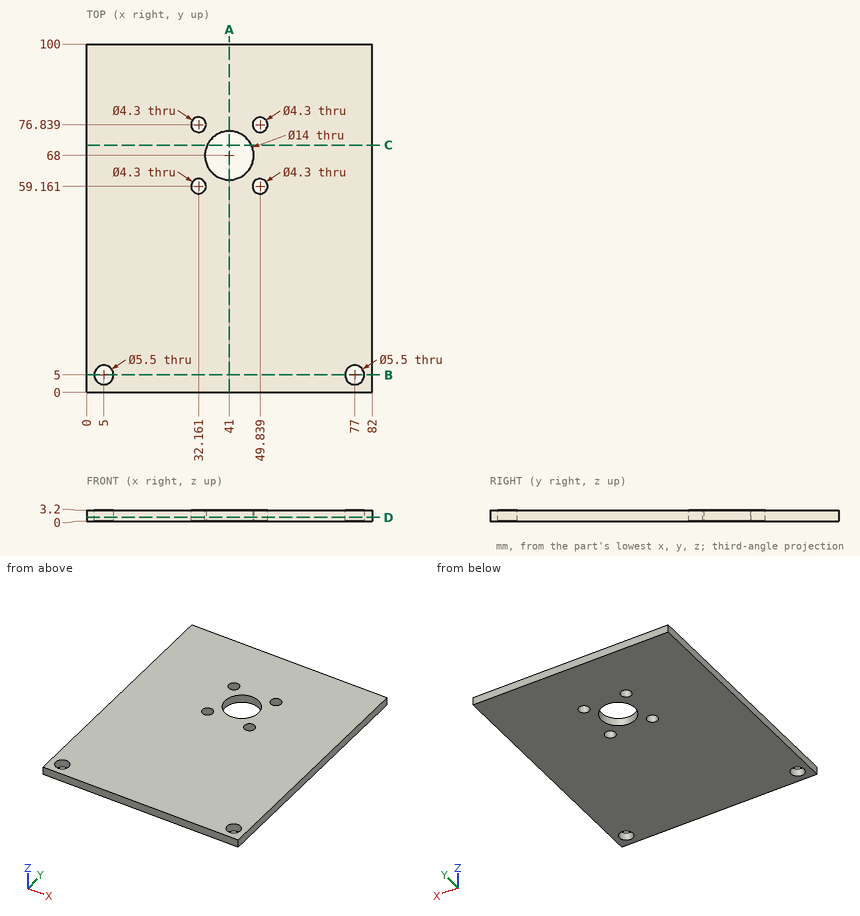
Can you work these out from the drawing? Everything is in mm from the part's minimum corner. Give positions to 0.01 mm unless a question says otherwise; leave off trailing zeros. Order: outer loops, then holes, each group sorted by start corner. A loop starts at its lowest first (then second) coordinate and runs counter-clockwise, first axis right, second up. Notation, with made-up numbers: (-38, 82.25) -> (-16, 82.25) arc R27 ccw to (-16, 114.25) -> close; hole circle Ø2 at (84.25, 34.25). An arc over 180 degrees is marked (long way). Return JSON: item names as keys, results as strings.
1. I need wall thicknesses on line 1 (X direction, y = 75.5, z = 2.25); line 2 (X direction, y = 6.5, z = 2.7) (1 decimal); line 3 (Y direction, x = 41, z = 1.5). Which ranges of each line are inside material? Lowest first, please. Write a range as from..to.
Answer list:
{"line 1": "x = 0..30.48, 33.84..48.16, 51.52..82", "line 2": "x = 0..2.7, 7.3..74.7, 79.3..82", "line 3": "y = 0..61, 75..100"}
2. Imagine slicing it at B-B on y = 5. List the corners of the cut face in (x, z) for me.
Answer list:
{"outline": "(0, 0) -> (2.25, 0) -> (2.25, 3.2) -> (0, 3.2) -> close; (7.75, 0) -> (74.25, 0) -> (74.25, 3.2) -> (7.75, 3.2) -> close; (79.75, 0) -> (82, 0) -> (82, 3.2) -> (79.75, 3.2) -> close"}
3. Imagine slicing it at C-C on y = 71. List the corners of the cut face in (x, z) for me, then the cut area to 3 significant figures.
Answer list:
{"outline": "(0, 0) -> (34.68, 0) -> (34.68, 3.2) -> (0, 3.2) -> close; (47.32, 0) -> (82, 0) -> (82, 3.2) -> (47.32, 3.2) -> close", "area": "222 mm2"}
4. Imagine slicing it at A-A on x = 41. List the corners of the cut face in (y, z) for me.
Answer list:
{"outline": "(0, 0) -> (61, 0) -> (61, 3.2) -> (0, 3.2) -> close; (75, 0) -> (100, 0) -> (100, 3.2) -> (75, 3.2) -> close"}
5. Imagine slicing it at D-D on z = 1.2. List the corners of the cut face in (x, y) for me, then the cut area to 3 significant figures.
Answer list:
{"outline": "(0, 0) -> (82, 0) -> (82, 100) -> (0, 100) -> close; hole circle Ø5.5 at (5, 5); hole circle Ø4.3 at (32.16, 59.16); hole circle Ø4.3 at (32.16, 76.84); hole circle Ø14 at (41, 68); hole circle Ø4.3 at (49.84, 59.16); hole circle Ø4.3 at (49.84, 76.84); hole circle Ø5.5 at (77, 5)", "area": "7,940 mm2"}
